Verification items for the finished model (mm, model axes). Face numbers are marked on the shaded views. A direction names the side the tool comes from. Coordinates: 2 decimals unless noted, no trailing zeros. Write each loop counter-clockwise with the first axis right and the second up, starting at its lowest first coordinate (ties: lowest second). Pieces come first, ordered by that corner, then holes. Notation, with made-up numbers: M 24,-5 L 48,-5 A27 cw 48,16 Z; hole C 25,78.5 d4. An arc over 180 degrees is marked long. One line per item, written item: value.
Autodesk Fusion 360 part; units mm, degrees
sketch "Sketch1" plane through (0, 0, 0) normal (0, 0, 1) x (1, 0, 0)
  line L0 (52, 8) -> (-52, 8)
  line L1 (-52, 8) -> (-52, -8)
  line L2 (-52, -8) -> (52, -8)
  line L3 (52, -8) -> (52, 8)
  line L4 (52, 8) -> (-52, -8) construction
  line L5 (-52, 8) -> (52, -8) construction
  circle A0 centre (-44, 0) radius 2.5
  line L6 (-38.2, 8) -> (-38.2, -8)
  line L7 (-35.2, 8) -> (-35.2, -8)
  line L8 (-31, 8) -> (-31, -8)
  line L9 (-28, 8) -> (-28, -8)
  line L10 (0, 1.75) -> (0, 22.5)
  line L11 (28, 8) -> (28, -8)
  line L12 (31, 8) -> (31, -8)
  line L13 (35.2, 8) -> (35.2, -8)
  line L14 (38.2, 8) -> (38.2, -8)
  circle A1 centre (44, 0) radius 2.5
  dimension "d1" = 104
  dimension "d2" = 16
  dimension "d3" = 5
  dimension "d4" = 8
  dimension "d6" = 3
  dimension "d7" = 31
  dimension "d8" = 3
  dimension "d9" = 4.2
extrude "Extrude1" add sketch "Sketch1" along normal blind 4
extrude "Extrude2" add sketch "Sketch1" along normal blind 12 contours L0 L2 L13 L14 | L0 L2 L11 L12 | L0 L2 L8 L9 | L0 L2 L6 L7
fillet "Fillet1" radius 8 4 edges at (-52, -8, 2) (-52, 8, 2) (52, 8, 2) (52, -8, 2)
fillet "Fillet1" radius 3 8 edges at (-36.7, -8, 12) (-36.7, 8, 12) (-29.5, -8, 12) (-29.5, 8, 12) (29.5, 8, 12) (29.5, -8, 12) (36.7, -8, 12) (36.7, 8, 12)
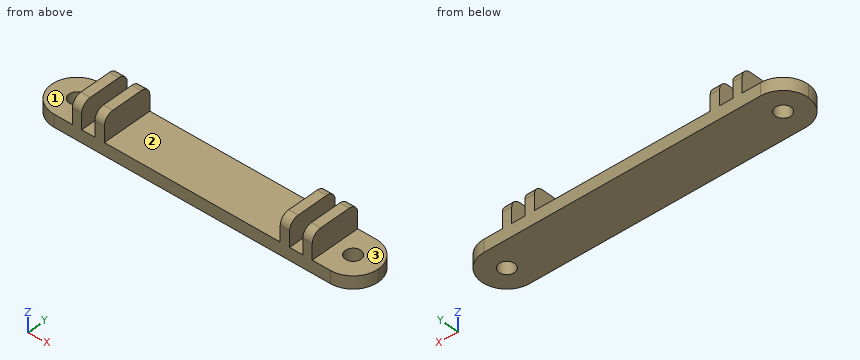
Item 1: Cross-section at B-B, the plane z = 1.5. Give the number of separate pieces and of enclosed holes in the cut face, and give its area (3 significant figures).
The answers:
separate pieces: 1
enclosed holes: 2
area: 1,570 mm²
Item 2: Go/stop test with flat-tipped pins: P1, Ø6.5, axis at y = 1, z = 8, coming from the +X side; P2, Ø1.3, axis at x = 33.5, y = 2.5, coming from the +Z side; P3, Ø4, axis at y = -0.5, z = 9, coming from the -X side; P4, Ø3, axis at x = 44, y = 0, coming from the -Z side. Record where each tip stops, or that it passes through.
The answers:
P1: stops at x = 38.2
P2: stops at z = 4
P3: stops at x = -38.2
P4: passes through
Item 3: Cross-section at D-D, the plane x = -21.5. Enter the section's corners in (y, z).
The answers:
outline: M -8,0 L 8,0 L 8,4 L -8,4 Z
Item 4: Cross-section at C-C, the plane y = 1. Enter the section's corners in (x, z), and give its area (3 significant figures).
The answers:
outline: M -51.94,0 L -46.29,0 L -46.29,4 L -51.94,4 Z; M -41.71,0 L 41.71,0 L 41.71,4 L 38.2,4 L 38.2,12 L 35.2,12 L 35.2,4 L 31,4 L 31,12 L 28,12 L 28,4 L -28,4 L -28,12 L -31,12 L -31,4 L -35.2,4 L -35.2,12 L -38.2,12 L -38.2,4 L -41.71,4 Z; M 46.29,0 L 51.94,0 L 51.94,4 L 46.29,4 Z
area: 475 mm²
Item 5: Cross-section at A-A, the plane z = 7.75. Enter the section's corners in (x, y), and give its area (3 significant figures).
The answers:
outline: M -38.2,-8 L -35.2,-8 L -35.2,8 L -38.2,8 Z; M -31,-8 L -28,-8 L -28,8 L -31,8 Z; M 28,-8 L 31,-8 L 31,8 L 28,8 Z; M 35.2,-8 L 38.2,-8 L 38.2,8 L 35.2,8 Z
area: 192 mm²
Item 6: Scan lines: line 1 (X direction, y = 3.5, z = 4.5); line 2 (Y direction, x = -44, z = 1.4); line 3 (Z direction, x = 24, y = 2.5). Record each from-to range of solid material in increasing order.
The answers:
line 1: x = -38.2 to -35.2, -31 to -28, 28 to 31, 35.2 to 38.2
line 2: y = -8 to -2.5, 2.5 to 8
line 3: z = 0 to 4
Item 7: Access from +Z, -Z, +X, -X, +Y, -Y to the whole of each face (thin tool, end or side, straight path). Record for the marked faces 1, 2 and 3.
The answers:
face 1: +Z, -X, +Y, -Y
face 2: +Z, +Y, -Y
face 3: +Z, +X, +Y, -Y
